The drawing under review shows one solid part. Ordinate dimensions are in mm from its lowest x, y, z. A direction names the side the tool comes from. Give positions to 0.01 mm unless a question says otherwise; leave off trailing zeros. Loops run counter-clockwise (first coordinate to the right, second up) from the corner with the lowest first, then second, coordinate; pieces in that order, holes last. Notation, with made-up numbers: (53, 81) - (110, 81) arc R16 ccw to (110, 98) - close; hole circle Ø7 at (15.25, -36). An arc over 180 degrees is marked (long way). One line per item, written item: value. Start each with the question number.
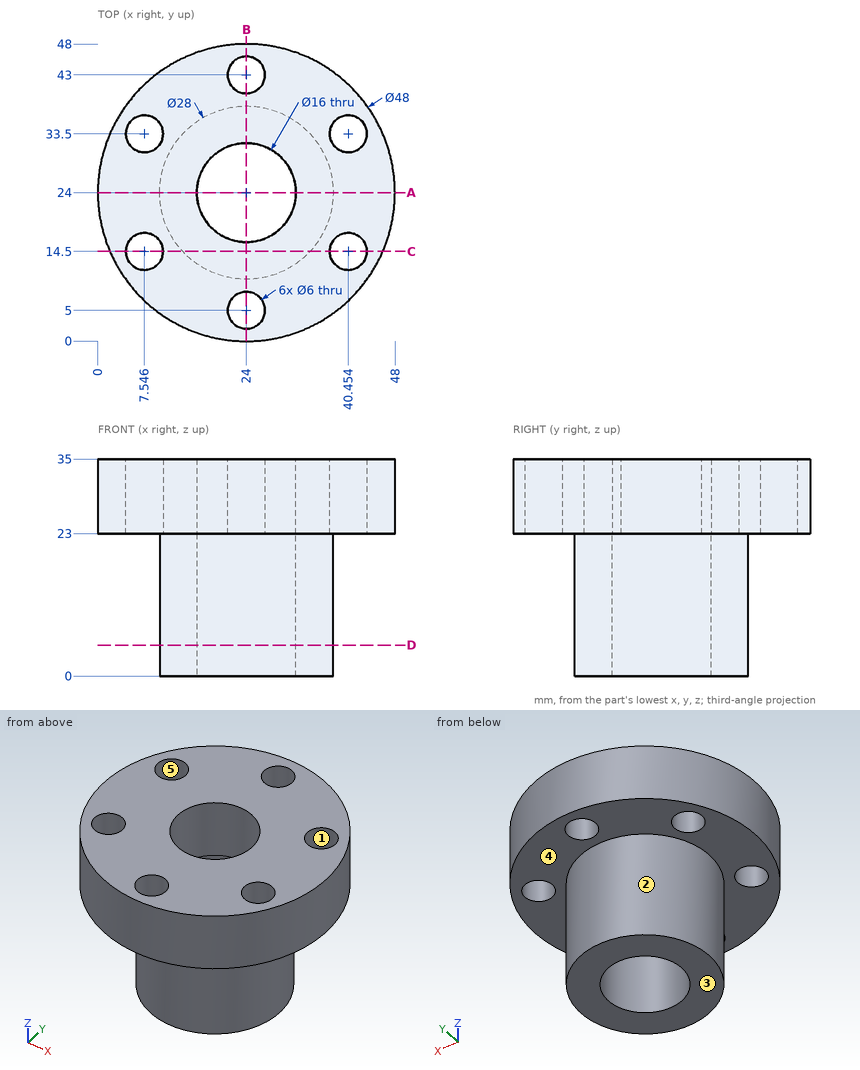
(1) Take a section at C-C on y = 14.5. State the section outline as (x, z) points (1 decimal), and give its area (3 significant figures).
(2) Take a section at D-D on z = 5. State the section outline as (x, y) points, and give its area (3 significant figures).
(3) Take a section at A-A on y = 24. State the section outline as (x, z) points.
(4) Draft analysis for pull direction Y (two halves, no side actions). For the marked faces 1, 2 and 3, state which applies: pulls with the +Y half, pulls with the -Y half, needs draft (parallel to the pull), parting line crosses it, or undercut.
(5) To check wall thickness, follow L1, parallel to Y at x = 24, z = 32.5; L2, parallel to Y at x = 24, z = 7; L3, parallel to Z at x = 15.5, y = 35.5. State the ranges of each line that lie inside material, in increasing order. Write a range as from..to.
(6) Machinability: for the marked faces 4 and 5, which of the approach directions +Z, -Z, +X, -X, +Y, -Y give a long, thin tool a straight path to every point of the face, cutting with its end or side? Answer none if there is none.
(7) Take a section at B-B on x = 24. State the section outline as (y, z) points.
(8) For pin 1 Ø2 at (x, z) = (6, 24.5) entering from +Y; pin 2 Ø1.5 at (y, z) = (14.5, 19) entering from +X; pin 3 Ø7 at (x, y) = (40.45, 33.5) entering from -Z; pin 4 Ø10 at (x, y) = (12, 36) entering from -Z, all flat-tipped, find the tip position at first contact; note any pin that passes through.
Here are the results:
1. outline: (2, 23) - (4.5, 23) - (4.5, 35) - (2, 35) - close; (10.5, 23) - (13.7, 23) - (13.7, 0) - (34.3, 0) - (34.3, 23) - (37.5, 23) - (37.5, 35) - (10.5, 35) - close; (43.5, 23) - (46, 23) - (46, 35) - (43.5, 35) - close
1. area: 858 mm²
2. outline: circle Ø28 at (24, 24); hole circle Ø16 at (24, 24)
2. area: 415 mm²
3. outline: (0, 23) - (10, 23) - (10, 0) - (16, 0) - (16, 35) - (0, 35) - close; (32, 0) - (38, 0) - (38, 23) - (48, 23) - (48, 35) - (32, 35) - close
4. face 1: undercut
4. face 2: parting line crosses it
4. face 3: needs draft
5. L1: 0..2, 8..16, 32..40, 46..48
5. L2: 10..16, 32..38
5. L3: 23..35
6. face 4: -Z
6. face 5: +Z, -Z
7. outline: (0, 23) - (2, 23) - (2, 35) - (0, 35) - close; (8, 23) - (10, 23) - (10, 0) - (16, 0) - (16, 35) - (8, 35) - close; (32, 0) - (38, 0) - (38, 23) - (40, 23) - (40, 35) - (32, 35) - close; (46, 23) - (48, 23) - (48, 35) - (46, 35) - close
8. pin 1: y = 40.94
8. pin 2: x = 34.93
8. pin 3: z = 23
8. pin 4: z = 0
